Design review of the part built by this model. Coordinates are the model's own, in mm. Face numbers are marked on the shaded views. A direction names the side the tool comes from. Round coordinates to 2 decimals unless told otherwise and drop trailing zeros. Write each loop counter-clockwise with the first axis right and the second up, starting at its lowest first coordinate (ties: lowest second). Pieces come first, ordered by that corner, then holes. Notation, with made-up numbers: (-39, 31) -> (13, 31) arc R7 cw to (13, 43) -> close; hole circle Ø3 at (-39, 78). An arc over 180 degrees is marked (long way). Write item = value, one per line. Start each with the question number.
Item 1: Add section D-D, the plane x = 87.5. State the section outline as (y, z) points.
Item 2: For pin 1 Ø4.5 at (x, z) = (106, 2) entering from -Y; pin 2 Ø5 at (x, y) = (7.5, -67.5) entering from -Z; pin 3 Ø6 at (x, y) = (87.5, -10.34) entering from -Z, all flat-tipped, find the tip position at first contact; note any pin that passes through.
Item 3: To check wall thickness, follow L1, parallel to X at y = -53, z = -29; L2, parallel to Y at x = 87.5, z = 2.95; L3, parallel to Z at x = 111, y = -43.5. State the ranges of each line that lie inside material, in increasing order.
Item 4: Add section B-B, the plane x = 131. State the section outline as (y, z) points, then the cut area to 3 significant figures.
Item 5: Add section C-C, the plane y = -34. State the section outline as (x, z) points.
Item 6: Machinability: for the marked faces 1 and 2, which of the approach directions +Z, -Z, +X, -X, +Y, -Y give a long, thin tool a straight path to every point of the face, cutting with its end or side? Answer none if there is none.
Item 7: Add section A-A, the plane z = -7. State the section outline as (x, y) points, then the cut area to 3 significant figures.
Item 8: Mouldability with a two-part tool opening along Z and no side actions: class the marked faces 3, 4 and 5 as released by +Z, released by -Z, zero draft, split by the parting line, or undercut.
from build123d import *

# Parameters (mm, degrees)
F0_W      = 3.2
F0_H      = 60
F0_W_2    = 168.6
F1_DEPTH  = 3
F2_DEPTH  = 37.2
F3_W      = 60
F3_H      = 3.2
F4_DEPTH  = 168.6
F5_W      = 15
F5_H      = 3
F6_DEPTH  = 15
F7_W      = 15
F7_H      = 3
F8_DEPTH  = 15
F9_R      = 2.25
F10_DEPTH = 25
F11_DEPTH = 1
F12_SIZE  = 2.5
F13_W     = 35.8230434358
F13_H     = 13.5607076809
F14_DEPTH = 175.001
F15_R     = 5
F16_DEPTH = 25
F17_R     = 7.49999
F18_DEPTH = 40.3


# Not quite as in the source:
# - a fillet or chamfer is up to 0.001 mm smaller than in the source, because OpenCascade refuses the exact size


with BuildPart() as f1:
    # F0 (on Top) → F1 (new body)
    with BuildSketch(Plane.XY):
        with Locations((1.6, -30)):
            Rectangle(F0_W, F0_H)
        with Locations((87.5, -30)):
            Rectangle(F0_W_2, F0_H)
        with Locations((173.4, -30)):
            Rectangle(F0_W, F0_H)
    extrude(amount=F1_DEPTH)

    # F0 (on Top) → F2 (join)
    with BuildSketch(Plane.XY):
        with Locations((1.6, -30)):
            Rectangle(F0_W, F0_H)
        with Locations((173.4, -30)):
            Rectangle(F0_W, F0_H)
    extrude(amount=-F2_DEPTH)

    # F3 (on face) → F4 (join, through all)
    with BuildSketch(Plane(origin=(171.8, 0, 0), x_dir=(0, -1, 0), z_dir=(-1, 0, 0))):
        with Locations((30, -35.6)):
            Rectangle(F3_W, F3_H)
    extrude(amount=F4_DEPTH)

    # F5 (on face) → F6 (join)
    with BuildSketch(Plane.XZ.offset(60)):
        with Locations((7.5, 1.5)):
            Rectangle(F5_W, F5_H)
        with Locations((167.5, 1.5)):
            Rectangle(F5_W, F5_H)
    extrude(amount=F6_DEPTH)

    # F7 (on face) → F8 (join)
    with BuildSketch(Plane(origin=(0, 0, 0), x_dir=(-1, 0, 0), z_dir=(0, 1, 0))):
        with Locations((-167.5, 1.5)):
            Rectangle(F7_W, F7_H)
        with Locations((-7.5, 1.5)):
            Rectangle(F7_W, F7_H)
    extrude(amount=F8_DEPTH)

    # F9 (on face) → F10 (cut)
    with BuildSketch(Plane.XY.offset(3)):
        with Locations((167.5, 7.5)):
            Circle(F9_R)
        with Locations((167.5, -67.5)):
            Circle(F9_R)
        with Locations((7.5, -67.5)):
            Circle(F9_R)
        with Locations((87.5, -10.3430738673)):
            Circle(F9_R)
    extrude(amount=-F10_DEPTH, mode=Mode.SUBTRACT)

    # F11 (add): a face of the model
    f11_faces = [f1.faces().sort_by_distance(p)[0] for p in [
        (87.3877644613, -29.9749671624, 3),
    ]]
    extrude(f11_faces, amount=F11_DEPTH)

    # F12
    f12_edges = [f1.edges().sort_by_distance(p)[0] for p in [
        (165.25, -67.5, 0),
        (165.25, 7.5, 0),
        (85.25, -10.343074, 0),
        (5.25, -67.5, 0),
    ]]
    chamfer(f12_edges, length=F12_SIZE)

    # F13 (on face) → F14 (cut, through all)
    with BuildSketch(Plane(origin=(0, 0, 0), x_dir=(0, -1, 0), z_dir=(-1, 0, 0))):
        with Locations((-17.9115217179, 6.7803538404)):
            Rectangle(F13_W, F13_H)
    extrude(amount=-F14_DEPTH, mode=Mode.SUBTRACT)

    # F15 (on face) → F16 (cut)
    with BuildSketch(Plane.XY.offset(-34)):
        with Locations((87.5478237867, -10.3831542656)):
            Circle(F15_R)
    extrude(amount=-F16_DEPTH, mode=Mode.SUBTRACT)

    # F17 (radius 7.5 in the source; OpenCascade refuses exactly that, so slightly less here)
    f17_edges = [f1.edges().sort_by_distance(p)[0] for p in [
        (15, -75, 2),
        (0, -75, 2),
        (160, -75, 2),
        (175, -75, 2),
    ]]
    fillet(f17_edges, radius=F17_R)

    # F18 (cut): a face of the model
    f18_faces = [f1.faces().sort_by_distance(p)[0] for p in [
        (87.5, -60, 2),
    ]]
    extrude(f18_faces, amount=-F18_DEPTH, mode=Mode.SUBTRACT)


solid = f1.part
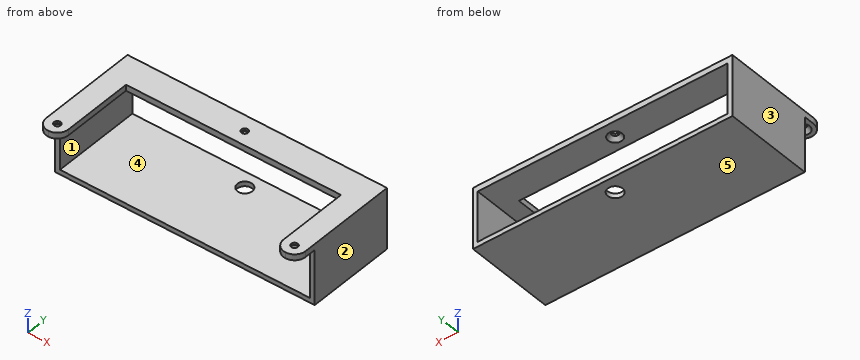
Result set:
q1.outline = (-60, -37.2) -> (-15.38, -37.2) -> (-15.38, -34) -> (-60, -34) -> close; (-19.7, 0) -> (-15.09, 0) -> (-12.59, 2.5) -> (-12.59, 4) -> (-19.7, 4) -> close; (-8.09, 2.5) -> (-5.59, 0) -> (0, 0) -> (0, 4) -> (-8.09, 4) -> close; (-5.38, -37.2) -> (0, -37.2) -> (0, -34) -> (-5.38, -34) -> close
q2.pin_1 = -19.7
q2.pin_2 = 2.25
q2.pin_3 = 1.75
q3.L1 = 0 to 3.2, 171.8 to 175
q3.L2 = -19.7 to -12.59, -8.09 to 0
q3.L3 = -37.2 to -34
q4.outline = (-60, -37.2) -> (0, -37.2) -> (0, -34) -> (-60, -34) -> close; (-19.7, 0) -> (0, 0) -> (0, 4) -> (-19.7, 4) -> close
q4.area = 271 mm²
q5.outline = (0, -37.2) -> (175, -37.2) -> (175, 4) -> (160, 4) -> (160, 0) -> (171.8, 0) -> (171.8, -34) -> (3.2, -34) -> (3.2, 0) -> (15, 0) -> (15, 4) -> (0, 4) -> close
q6.face_1 = +Y, -Y
q6.face_2 = +Z, -Z, +X, +Y, -Y
q7.outline = (0, -60) -> (3.2, -60) -> (3.2, 0) -> (0, 0) -> close; (171.8, -60) -> (175, -60) -> (175, 0) -> (171.8, 0) -> close
q7.area = 384 mm²
q8.face_3 = zero draft
q8.face_4 = undercut
q8.face_5 = released by -Z
